For this review, take the finished solid that the model builds, in its own axes (mm). Face numbers are marked on the shaded views. A direction names the side the tool comes from. Coordinates: 2 decimals unless noted, no trailing zeros. Loops run counter-clockwise (first coordinate to the right, second up) from the corner with the lowest first, then second, coordinate; pieces in that order, holes last. Notation, with made-up numbers: M -17,65.5 L -2,65.5 A21 cw -2,99.5 Z; hole C 39,89.5 d10. An arc over 180 degrees is marked long. Use one line per item in the form item = value.
```python
from build123d import *

# Parameters (mm, degrees)
SKETCH2_R           = 17.604244625
BOSS_EXTRUDE1_DEPTH = 2
SKETCH3_R           = 18.437955777
BOSS_EXTRUDE2_DEPTH = 2


with BuildPart() as part:
    # Sketch1 → Revolve-Thin2 (revolve)
    with BuildSketch(Plane.XY):
        Polygon((-49.689400151, 17.604244625), (-38.615762403, 17.604244625), (-5.678788589, 7.666364595), (9.653940601, 7.666364595), (41.968714147, 18.437955777), (53.905013296, 18.437955777), (53.905013296, 16.437955777), (42.293269467, 16.437955777), (9.978495921, 5.666364595), (-5.973941532, 5.666364595), (-38.910915347, 15.604244625), (-49.689400151, 15.604244625), align=None)
    revolve(axis=Axis((0, 0, 0), (-1, 0, 0)))

    # Sketch2 → Boss-Extrude1 (add)
    with BuildSketch(Plane.ZY.offset(49.689400151)):
        Circle(SKETCH2_R)
    extrude(amount=BOSS_EXTRUDE1_DEPTH)

    # Sketch3 → Boss-Extrude2 (add)
    with BuildSketch(Plane(origin=(53.905013296, 0, 0), x_dir=(0, 0, -1), z_dir=(1, 0, 0))):
        Circle(SKETCH3_R)
    extrude(amount=BOSS_EXTRUDE2_DEPTH)


solid = part.part
```
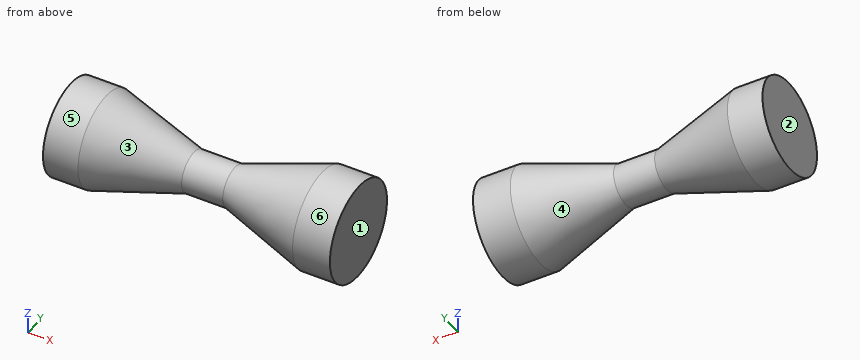
1. Draft analysis for pull direction X (two halves, no side actions). For the marked faces 1, 2 and 3, state which applies: +X half, -X half, draft (parallel to the pull), parting line (faces both ways), or undercut.
Computed values:
face_1 = +X half
face_2 = -X half
face_3 = undercut
2. Consider section A-A on y = 0. Write out the cut boundary in (x, z).
Computed values:
outline = M -51.69,-17.6 L -38.62,-17.6 L -5.68,-7.67 L 9.65,-7.67 L 41.97,-18.44 L 55.91,-18.44 L 55.91,18.44 L 41.97,18.44 L 9.65,7.67 L -5.68,7.67 L -38.62,17.6 L -51.69,17.6 Z; hole M -49.69,-15.6 L -38.91,-15.6 L -5.97,-5.67 L 9.98,-5.67 L 42.29,-16.44 L 53.91,-16.44 L 53.91,16.44 L 42.29,16.44 L 9.98,5.67 L -5.97,5.67 L -38.91,15.6 L -49.69,15.6 Z
3. Tool access review of the marked faces 4, 5 and 6: name each direction out of +Z, -Z, +X, -X, +Y, -Y from which nothing blocks a thin tool from reaching the whole face with its end or side.
Computed values:
face_4 = none
face_5 = -X
face_6 = +X, -X
4. Consider section C-C on x = -2. Write out the cut boundary in (y, z), plus the area to 3 significant figures.
Computed values:
outline = C 0,0 d15.33; hole C 0,0 d11.33
area = 83.8 mm2
5. Wall thickness on line 1 along Z through (x, y) = (7.25, 0); line 2 along X through (y, z) = (-7, -6): over which ranges is each line inside the solid? List them lowest first. Write a range as from..to.
Computed values:
line_1 = -7.67..-5.67, 5.67..7.67
line_2 = -51.69..-49.69, -17.75..-10.83, 14.31..20.64, 53.91..55.91
6. Consider section D-D on z = -11. State how many separate pieces and enclosed holes the cut face has, plus the area to 3 significant figures.
Computed values:
separate_pieces = 2
enclosed_holes = 2
area = 577 mm2
7. For pin 1 Ø4 at (x, z) = (-25.5, -9) entering from -Y; pin 2 Ø6 at (x, y) = (0.5, -3) entering from -Z; pin 3 Ø10 at (x, z) = (-18, -7) entering from +Y, all flat-tipped, find the tip position at first contact; note any pin that passes through.
Computed values:
pin_1 = -11.91
pin_2 = -7.67
pin_3 = 11.96
